```python
from build123d import *

# Parameters (mm, degrees)
F0_W     = 73.66
F0_H     = 48.26
F0_R     = 2.1082
F0_R_2   = 2.7051
F1_DEPTH = 3.175
F2_SIZE  = 2.54


with BuildPart() as f1:
    # F0 (on Top) → F1 (new body)
    with BuildSketch(Plane.XY):
        Rectangle(F0_W, F0_H)
        with Locations((28.321, -13.335)):
            Circle(F0_R, mode=Mode.SUBTRACT)
        with Locations((-25.4, 0)):
            Circle(F0_R_2, mode=Mode.SUBTRACT)
        with Locations((-12.7, 0)):
            Circle(F0_R_2, mode=Mode.SUBTRACT)
        with Locations((-28.321, 13.335)):
            Circle(F0_R, mode=Mode.SUBTRACT)
        with Locations((12.7, 0)):
            Circle(F0_R_2, mode=Mode.SUBTRACT)
        with Locations((25.4, 0)):
            Circle(F0_R_2, mode=Mode.SUBTRACT)
    extrude(amount=F1_DEPTH)

    # F2
    f2_edges = [f1.edges().sort_by_distance(p)[0] for p in [
        (-30.4292, 13.335, 3.175),
        (26.2128, -13.335, 3.175),
    ]]
    chamfer(f2_edges, length=F2_SIZE)


solid = f1.part
```
Geometry check sheet. Reference: the model listing, model coordinates, mm. Give positions to 0.01 mm unless a question says otherwise; leave off trailing zeros. Order: outer loops, then holes, each group sorted by start corner. A loop starts at its lowest first (then second) coordinate and runs counter-clockwise, first axis right, second up.
1. Section check C-C, the plane z = 1.45. Enter the section's corners in (x, y) (3 decimals).
2. Thickness scan on L1, parallel to Y at x = 12.7, z = 1.55; L2, parallel to Y at x = 24.5, z = 2.95; L3, parallel to Y at x = -26, z = 2. Record the ranges inside material, lowest first.
3. Gauge pin test, flat ends, axial feed: pin 1 Ø3.5 at (x, y) = (28.321, -13.335) entering from +Z; pin 2 Ø5.5 at (x, y) = (-28.321, 13.335) entering from +Z. Record the tip position at first contact, or that the pin passes through.
4. Section check B-B, the plane y = 0. Enter the section's corners in (x, z) (3 decimals).
5. Section check A-A, the plane x = 12.7. Enter the section's corners in (y, z) (3 decimals), and give its area (3 significant figures).
6. Release check for a two-part mould opening along X. For faces 1 (the face through (-1, -24.13, 2)), 2 (the face through (-36.83, 0, 2)), 3 (the face through (-28.102, 0.119, 1.565)) record: pulls with the +X half, pulls with the -X half, needs draft (parallel to the pull), parting line crosses it, or undercut.
Values follow:
1. outline: (-36.83, -24.13) - (36.83, -24.13) - (36.83, 24.13) - (-36.83, 24.13) - close; hole circle Ø5.846 at (-28.321, 13.335); hole circle Ø5.41 at (-25.4, 0); hole circle Ø5.41 at (-12.7, 0); hole circle Ø5.41 at (12.7, 0); hole circle Ø5.41 at (25.4, 0); hole circle Ø5.846 at (28.321, -13.335)
2. L1: y = -24.13 to -2.71, 2.71 to 24.13
2. L2: y = -24.13 to -15.56, -11.11 to -2.55, 2.55 to 24.13
2. L3: y = -24.13 to -2.64, 2.64 to 10.75, 15.92 to 24.13
3. pin 1: passes through
3. pin 2: stops at z = 1.28
4. outline: (-36.83, 0) - (-28.105, 0) - (-28.105, 3.175) - (-36.83, 3.175) - close; (-22.695, 0) - (-15.405, 0) - (-15.405, 3.175) - (-22.695, 3.175) - close; (-9.995, 0) - (9.995, 0) - (9.995, 3.175) - (-9.995, 3.175) - close; (15.405, 0) - (22.695, 0) - (22.695, 3.175) - (15.405, 3.175) - close; (28.105, 0) - (36.83, 0) - (36.83, 3.175) - (28.105, 3.175) - close
5. outline: (-24.13, 0) - (-2.705, 0) - (-2.705, 3.175) - (-24.13, 3.175) - close; (2.705, 0) - (24.13, 0) - (24.13, 3.175) - (2.705, 3.175) - close
5. area: 136 mm2
6. face 1: needs draft
6. face 2: pulls with the -X half
6. face 3: undercut
